from build123d import *

# Parameters (mm, degrees)
F2_DEPTH = 444.5
F3_ANGLE = 90
F5_D     = 7.9375


# Not quite as in the source:
# - a variable given as a bare number and used for a length is read in inches; the dataset says mm whatever the document's units were


with BuildPart() as f2:
    # F0 (on Top) → F2 (new body)
    with BuildSketch(Plane.XY):
        with BuildLine():
            Line((-12.573, -15.875), (12.573, -15.875))
            ThreePointArc((12.573, -15.875), (14.9078665915, -14.9078665915), (15.875, -12.573))
            Line((15.875, -12.573), (15.875, 12.573))
            ThreePointArc((15.875, 12.573), (14.9078665915, 14.9078665915), (12.573, 15.875))
            Line((12.573, 15.875), (-12.573, 15.875))
            ThreePointArc((-12.573, 15.875), (-14.9078665915, 14.9078665915), (-15.875, 12.573))
            Line((-15.875, 12.573), (-15.875, -12.573))
            ThreePointArc((-15.875, -12.573), (-14.9078665915, -14.9078665915), (-12.573, -15.875))
        make_face()
        with BuildLine():
            Line((-12.573, 14.224), (12.573, 14.224))
            ThreePointArc((12.573, 14.224), (13.7404332957, 13.7404332957), (14.224, 12.573))
            Line((14.224, 12.573), (14.224, -12.573))
            ThreePointArc((14.224, -12.573), (13.7404332957, -13.7404332957), (12.573, -14.224))
            Line((12.573, -14.224), (-12.573, -14.224))
            ThreePointArc((-12.573, -14.224), (-13.7404332957, -13.7404332957), (-14.224, -12.573))
            Line((-14.224, -12.573), (-14.224, 12.573))
            ThreePointArc((-14.224, 12.573), (-13.7404332957, 13.7404332957), (-12.573, 14.224))
        make_face(mode=Mode.SUBTRACT)
    extrude(amount=F2_DEPTH)


with BuildPart() as f2_1:
    # F3: moved
    add(f2.part.rotate(Axis((-15.875, 0, 444.5), (0, 1, 0)), F3_ANGLE))

    # F5 (through all)
    with Locations(Plane.XY.offset(444.5)):
        with Locations((-365.125, 0), (-111.125, 0)):
            Hole(F5_D / 2)


solid = f2_1.part
Work out the finished part from the listing and answer in its coordinate system (mm). A direction names the side the tool comes from. Round coordinates to 2 decimals unless told otherwise and drop trailing zeros. Write each loop counter-clockwise with the first axis right and the second up, starting at its lowest first coordinate (ties: lowest second). Pieces come first, ordered by that corner, then holes. Notation, with made-up numbers: M 35.25,19 L 47.25,19 A15 cw 47.25,40 Z; hole C 85,18.5 d2. An arc over 180 degrees is marked long. Use a Markdown table: item, result.
1) The part is cut by section A-A on z = 425.5. Give the vertices of the cut face in (x, y) (3 decimals).
Taken from the geometry:
| item | result |
|---|---|
| outline | M -460.375,-15.875 L -15.875,-15.875 L -15.875,-14.224 L -460.375,-14.224 Z; M -460.375,14.224 L -15.875,14.224 L -15.875,15.875 L -460.375,15.875 Z |
2) A flat-ended cylindrical pin translates along its axis: pin 1 (10.5 mm diameter, centred on x = -365.125, y = 0, fed in from -Z). Find the tip coordinate at first contact, or state that the pin passes through.
Taken from the geometry:
| item | result |
|---|---|
| pin 1 | stops at z = 412.75 |
3) Consider line 1 (Y direction, x = -338.5, z = 430.5) (3 decimals); line 2 (Z direction, x = -167.5, y = -1). Determine where each line is inside the solid, lowest interval first. Write a range as [from, to].
Taken from the geometry:
| item | result |
|---|---|
| line 1 | y = [-15.875, -14.224], [14.224, 15.875] |
| line 2 | z = [412.75, 414.4], [442.85, 444.5] |
4) The part is cut by section C-C on x = -340. Give the vertices of the cut face in (y, z) (3 decimals).
Taken from the geometry:
| item | result |
|---|---|
| outline | M -15.875,416.052 A3.302 ccw -12.573,412.75 L 12.573,412.75 A3.302 ccw 15.875,416.052 L 15.875,441.198 A3.302 ccw 12.573,444.5 L -12.573,444.5 A3.302 ccw -15.875,441.198 Z; hole M -14.224,416.052 A1.651 ccw -12.573,414.401 L 12.573,414.401 A1.651 ccw 14.224,416.052 L 14.224,441.198 A1.651 ccw 12.573,442.849 L -12.573,442.849 A1.651 ccw -14.224,441.198 Z |
5) Determine the mould class of faces 3 (the face through (-114.91, 1.19, 413.56)), 4 (the face through (-241, 0, 412.75)), 5 (the face through (-241, 0, 414.401)), 6 (the face through (-241, 0, 444.5)) for opening direction Z: pulls with the +Z half, pulls with the -Z half, needs draft (parallel to the pull), parting line crosses it, or undercut.
Taken from the geometry:
| item | result |
|---|---|
| face 3 | needs draft |
| face 4 | pulls with the -Z half |
| face 5 | undercut |
| face 6 | pulls with the +Z half |
6) Which of the six approach directions +Z, -Z, +X, -X, +Y, -Y give full straight-line access (tool end or side, diameter ignored) to faces 1 (the face through (-241, 0, 442.849)), 2 (the face through (-241, -15.875, 429))?
Taken from the geometry:
| item | result |
|---|---|
| face 1 | +X, -X |
| face 2 | +Z, -Z, +X, -X, -Y |
7) The part is cut by section B-B on y = 0. Give the vertices of the cut face in (x, z) (3 decimals).
Taken from the geometry:
| item | result |
|---|---|
| outline | M -460.375,412.75 L -369.094,412.75 L -369.094,414.401 L -460.375,414.401 Z; M -460.375,442.849 L -369.094,442.849 L -369.094,444.5 L -460.375,444.5 Z; M -361.156,412.75 L -115.094,412.75 L -115.094,414.401 L -361.156,414.401 Z; M -361.156,442.849 L -115.094,442.849 L -115.094,444.5 L -361.156,444.5 Z; M -107.156,412.75 L -15.875,412.75 L -15.875,414.401 L -107.156,414.401 Z; M -107.156,442.849 L -15.875,442.849 L -15.875,444.5 L -107.156,444.5 Z |
